Source: CAD feature listing. Evaluate the final solid. Frame: model axes, mm. Face numbers are marked on the shaded views. Coordinates: 2 decimals unless noted, no trailing zeros. Loops run counter-clockwise (first coordinate to the right, second up) from the corner with the lowest first, then second, coordinate; pieces in that order, holes last.
from build123d import *

# Parameters (mm, degrees)
BOSS_EXTRUDE1_DEPTH = 12.7
SKETCH2_W           = 28.575
SKETCH2_H           = 20.955
BOSS_EXTRUDE2_DEPTH = 6.35
SKETCH2_2_W         = 28.575
SKETCH2_2_H         = 20.955
BOSS_EXTRUDE3_DEPTH = 5.08
SKETCH3_W           = 12.7
SKETCH3_H           = 6.35
CUT_EXTRUDE1_DEPTH  = 5.08
SKETCH4_R           = 1.524
CUT_EXTRUDE2_DEPTH  = 6.35
SKETCH6_R           = 2
BOSS_EXTRUDE4_DEPTH = 5


with BuildPart() as part:
    # Sketch1 → Boss-Extrude1 (new body)
    with BuildSketch(Plane(origin=(0, 0, 0), x_dir=(1, 0, 0), z_dir=(0, 1, 0))):
        with BuildLine():
            Line((-45.903249768, -53.250574222), (-42.783043149, -52.66326199))
            ThreePointArc((-42.783043149, -52.66326199), (0, 0), (44.879778188, -50.888244756))
            Line((44.879778188, -50.888244756), (48.021201665, -51.348770042))
            ThreePointArc((48.021201665, -51.348770042), (-0.064274965, 3.174349339), (-45.903249768, -53.250574222))
        make_face()
    extrude(amount=BOSS_EXTRUDE1_DEPTH)

    # Sketch2 → Boss-Extrude2 (add)
    with BuildSketch(Plane.XY):
        with Locations((0, 10.4775)):
            Rectangle(SKETCH2_W, SKETCH2_H)
    extrude(amount=-BOSS_EXTRUDE2_DEPTH)

    # Sketch2_2 → Boss-Extrude3 (add)
    with BuildSketch(Plane.XY):
        with Locations((0, 10.4775)):
            Rectangle(SKETCH2_2_W, SKETCH2_2_H)
    extrude(amount=-BOSS_EXTRUDE3_DEPTH)

    # Sketch3 → Cut-Extrude1 (cut)
    with BuildSketch(Plane(origin=(0, 0, -6.35), x_dir=(-1, 0, 0), z_dir=(0, 0, -1))):
        with Locations((0, 17.78)):
            Rectangle(SKETCH3_W, SKETCH3_H)
    extrude(amount=-CUT_EXTRUDE1_DEPTH, mode=Mode.SUBTRACT)

    # Sketch4 → Cut-Extrude2 (cut)
    with BuildSketch(Plane(origin=(0, 0, -6.35), x_dir=(-1, 0, 0), z_dir=(0, 0, -1))):
        with Locations((-10.16, 4.1275)):
            Circle(SKETCH4_R)
        with Locations((-10.16, 16.8275)):
            Circle(SKETCH4_R)
        with Locations((10.16, 4.1275)):
            Circle(SKETCH4_R)
        with Locations((10.16, 16.8275)):
            Circle(SKETCH4_R)
    extrude(amount=-CUT_EXTRUDE2_DEPTH, mode=Mode.SUBTRACT)

    # Sketch6 → Boss-Extrude4 (add)
    with BuildSketch(Plane(origin=(0, 0, 0), x_dir=(1, 0, 0), z_dir=(0, 1, 0))):
        Polygon((23.618693952, -0.791157312), (23.618693952, -2.892477036), (17.618693952, -2.892477036), (17.618693952, 46.708842688), (17.618693952, 53.708842688), (54, 53.708842688), (54, 46.708842688), (23.618693952, 46.708842688), (23.618693952, 6.208842688), (54, 6.208842688), (54, -0.791157312), (38.224238065, -14.85997386), (34.870951122, -11.062681088), (47, -0.791157312), align=None)
        with Locations((50.5, 3.708842688)):
            Circle(SKETCH6_R, mode=Mode.SUBTRACT)
        with Locations((28.5, 3.708842688)):
            Circle(SKETCH6_R, mode=Mode.SUBTRACT)
        with Locations((28.5, 50.208842688)):
            Circle(SKETCH6_R, mode=Mode.SUBTRACT)
        with Locations((50.5, 50.208842688)):
            Circle(SKETCH6_R, mode=Mode.SUBTRACT)
    extrude(amount=BOSS_EXTRUDE4_DEPTH)


solid = part.part
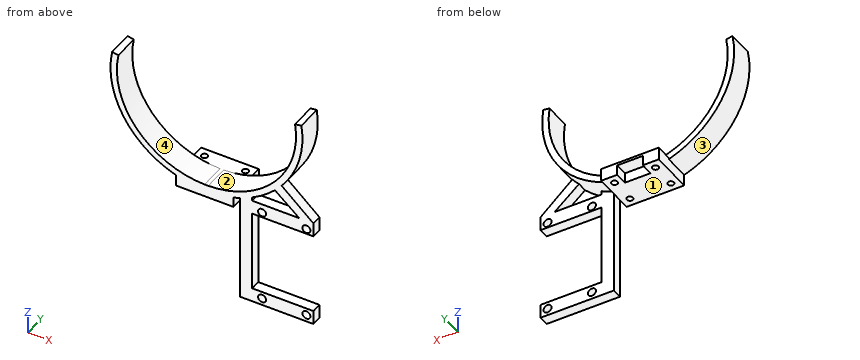
Q1. Section D-D, the plane x = 28.5. Return the cut outline in (y, z), plus the area to 3 significant figures.
Q2. Contact query for flat-ended pins moving along their axis: pin 1 Ø2.5 at (x, z) = (50.5, -50.21) entering from -Y; pin 2 Ø1.5 at (x, y) = (3.5, 8.5) entering from -Z; pin 3 Ø4 at (y, z) = (1.5, -38.5) entering from -X; pin 4 Ø12 at (x, z) = (14, -24.5) entering from +Y. Output: stop coordinate, or through.
Q3. Line query: line 1 along Y through (x, z) = (10.16, -3) (1 decimal); line 2 along Y through (x, z) = (-10, -2) (3 decimals); line 3 along Z through (x, y) = (37.5, 4.75). Output: solid intervals per line, ascending.
Q4. Section C-C, the plane z = 12.5. Return the cut outline in (x, y).
Q5. Draft query along X for the marked faces 1, 2, 3 and 4. Return one class per face: +X half, -X half, draft (parallel to the pull), parting line (faces both ways), or undercut.
Derived:
1. outline: (0, -53.71) - (5, -53.71) - (5, -52.21) - (0, -52.21) - close; (0, -48.21) - (5, -48.21) - (5, -46.71) - (0, -46.71) - close; (0, -6.21) - (5, -6.21) - (5, -5.71) - (0, -5.71) - close; (0, -1.71) - (5, -1.71) - (5, 0.79) - (0, 0.79) - close; (0, 5.63) - (12.7, 5.63) - (12.7, 9.6) - (0, 9.6) - close
1. area: 80.4 mm2
2. pin 1: passes through
2. pin 2: stops at z = -6.35
2. pin 3: stops at x = 17.62
2. pin 4: stops at y = 5
3. line 1: y = 0 to 2.6, 5.7 to 15.3, 18.4 to 21
3. line 2: y = 0 to 2.612, 5.643 to 15.312, 18.343 to 20.955
3. line 3: z = -53.71 to -46.71, -6.21 to 0.79, 8.84 to 19.22
4. outline: (-34.43, 0) - (-30.01, 0) - (-30.01, 12.7) - (-34.43, 12.7) - close; (31.81, 0) - (40.87, 0) - (40.87, 5) - (36.23, 5) - (36.23, 12.7) - (31.81, 12.7) - close
5. face 1: draft
5. face 2: undercut
5. face 3: -X half
5. face 4: undercut
